Verification items for the finished model (mm, model axes). Coordinates: 2 decimals unless noted, no trailing zeros. Loops run counter-clockwise (first coordinate to the right, second up) from the corner with the lowest first, then second, coordinate; pieces in that order, holes last. Notation, with made-up numbers: (5, 7) - (61, 7) arc R14 cw to (61, 13) - close; hole circle Ø5 at (54, 65). An arc over 180 degrees is marked (long way). One line per item, written item: value. Start each with the question number.
(1) Section check C-C (x = -45.5). Record the boundary of the cut face in (y, z).
(2) Thickness scan on probe 1 along Z at (x, y) = (155.5, 0); probe 2 along X at (y, z) = (3, 2.25); probe 3 along X at (y, z) = (2, 1.75). Record the ranges inside material, lowest first. Write a range as [from, to].
(3) Gauge pin test, flat ends, axial feed: P1, Ø1, axis at x = 136, z = -2, coming from the -Y side; P2, Ø7, axis at y = -0.5, z = 1, coming from the +X side; P3, Ø1, axis at y = 1, z = 1, coming from the -X side; P4, Ø2, axis at x = -38.5, z = -4.5, coming from the -Y side. Record the tip position at first contact, or that the pin passes through.
(4) Section check A-A (z = 0). Record the boundary of the cut face in (x, y).
(5) Section check D-D (x = 26.5). Record the boundary of the cut face in (y, z).
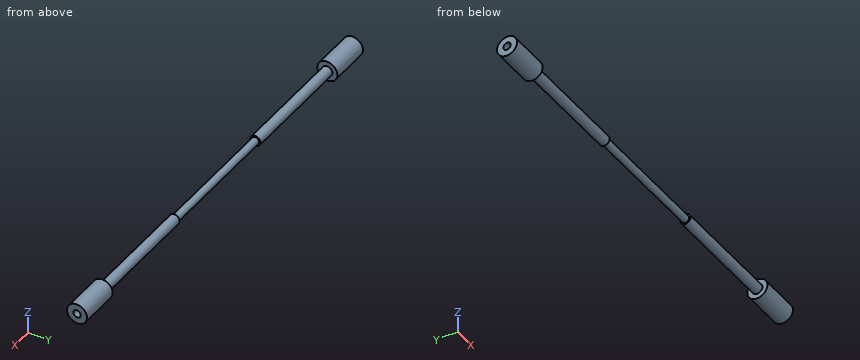
```python
from build123d import *

# Parameters (mm, degrees)
F0_R      = 2.3622
F1_DEPTH  = 105.39984
F3_R      = 3.2512
F4_DEPTH  = 96.52508
F6_R      = 3.2512
F7_DEPTH  = 96.52508
F8_R      = 6.35
F8_R_2    = 3.2512
F9_DEPTH  = 25.4
F10_R     = 2.3622
F11_DEPTH = 50.8
F12_R     = 6.35
F12_R_2   = 3.2512
F13_DEPTH = 25.4
F14_R     = 2.3622
F15_DEPTH = 50.8


with BuildPart() as f1:
    # F0 (on Right) → F1 (new body)
    with BuildSketch(Plane.YZ):
        Circle(F0_R)
    extrude(amount=F1_DEPTH)

    # F3 (on offset) → F4 (join)
    with BuildSketch(Plane.YZ.offset(12.7)):
        Circle(F3_R)
    extrude(amount=-F4_DEPTH)

    # F6 (on offset) → F7 (join)
    with BuildSketch(Plane.YZ.offset(92.69984)):
        Circle(F6_R)
    extrude(amount=F7_DEPTH)

    # F8 (on face) → F9 (join)
    with BuildSketch(Plane(origin=(-83.82508, 0, 0), x_dir=(0, -1, 0), z_dir=(-1, 0, 0))):
        Circle(F8_R)
        Circle(F8_R_2, mode=Mode.SUBTRACT)
    extrude(amount=-F9_DEPTH)

    # F10 (on face) → F11 (cut)
    with BuildSketch(Plane(origin=(-83.82508, 0, 0), x_dir=(0, -1, 0), z_dir=(-1, 0, 0))):
        Circle(F10_R)
    extrude(amount=-F11_DEPTH, mode=Mode.SUBTRACT)

    # F12 (on face) → F13 (join)
    with BuildSketch(Plane.YZ.offset(189.22492)):
        Circle(F12_R)
        Circle(F12_R_2, mode=Mode.SUBTRACT)
    extrude(amount=-F13_DEPTH)

    # F14 (on face) → F15 (cut)
    with BuildSketch(Plane.YZ.offset(189.22492)):
        Circle(F14_R)
    extrude(amount=-F15_DEPTH, mode=Mode.SUBTRACT)


solid = f1.part
```
Responses:
1. outline: circle Ø6.5 at (0, 0); hole circle Ø4.72 at (0, 0)
2. probe 1: z = [-3.25, -2.36], [2.36, 3.25]
2. probe 2: x = [-83.83, -58.43], [163.82, 189.22]
2. probe 3: x = [-83.83, 12.7], [92.7, 189.22]
3. P1: stops at y = -2.88
3. P2: stops at x = 189.22
3. P3: stops at x = -33.03
3. P4: passes through
4. outline: (-83.83, -6.35) - (-58.43, -6.35) - (-58.43, -3.25) - (12.7, -3.25) - (12.7, -2.36) - (92.7, -2.36) - (92.7, -3.25) - (163.82, -3.25) - (163.82, -6.35) - (189.22, -6.35) - (189.22, -2.36) - (138.42, -2.36) - (138.42, 2.36) - (189.22, 2.36) - (189.22, 6.35) - (163.82, 6.35) - (163.82, 3.25) - (92.7, 3.25) - (92.7, 2.36) - (12.7, 2.36) - (12.7, 3.25) - (-58.43, 3.25) - (-58.43, 6.35) - (-83.83, 6.35) - (-83.83, 2.36) - (-33.03, 2.36) - (-33.03, -2.36) - (-83.83, -2.36) - close
5. outline: circle Ø4.72 at (0, 0)
